Model file for the job. Use its own axes, mm. Face numbers are marked on the shaded views. A direction names the side the tool comes from. Round coordinates to 2 decimals unless told otherwise and drop trailing zeros. Loops run counter-clockwise (first coordinate to the right, second up) from the corner with the lowest first, then second, coordinate; pieces in that order, holes last. Notation, with made-up numbers: (60, 18) -> (112, 18) arc R17 ccw to (112, 51) -> close; hole circle Ø11 at (-7, -21). An arc over 180 degrees is marked (long way). Use a Markdown table: item, result.
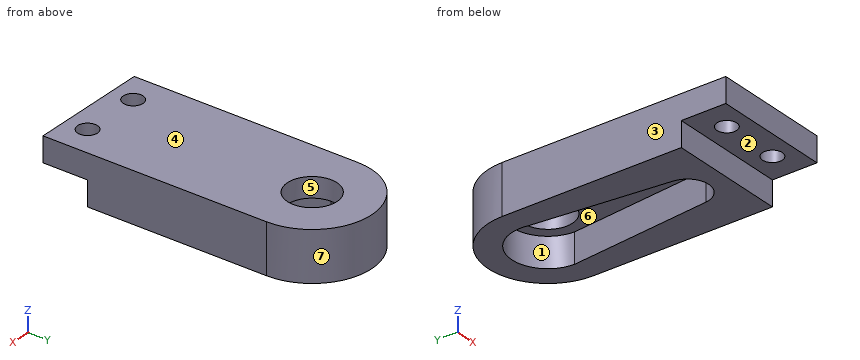
from build123d import *

# Parameters (mm, degrees)
SKETCH1_W           = 11.999998241
SKETCH1_H           = 22.605046118
BOSS_EXTRUDE1_DEPTH = 5
BOSS_EXTRUDE2_DEPTH = 5
SKETCH4_R           = 2.5
CUT_EXTRUDE3_DEPTH  = 5
CUT_EXTRUDE7_DEPTH  = 3
SKETCH10_W          = 11.999998241
SKETCH10_H          = 4.5
CUT_EXTRUDE8_DEPTH  = 2.5
SKETCH12_R          = 1
CUT_EXTRUDE9_DEPTH  = 5


with BuildPart() as part:
    # Sketch1 → Boss-Extrude1 (new body)
    with BuildSketch(Plane.XY):
        with Locations((-37.429383025, 291.690953332)):
            Rectangle(SKETCH1_W, SKETCH1_H)
    extrude(amount=BOSS_EXTRUDE1_DEPTH)

    # Sketch3 → Boss-Extrude2 (add)
    with BuildSketch(Plane.XY):
        with BuildLine():
            Line((-31.429383904, 302.993476391), (-43.429382145, 302.993476391))
            ThreePointArc((-43.429382145, 302.993476391), (-37.429383025, 308.993475512), (-31.429383904, 302.993476391))
        make_face()
    extrude(amount=BOSS_EXTRUDE2_DEPTH)

    # Sketch4 → Cut-Extrude3 (cut)
    with BuildSketch(Plane.XY):
        with Locations((-37.429383025, 302.993476391)):
            Circle(SKETCH4_R)
    extrude(amount=CUT_EXTRUDE3_DEPTH, mode=Mode.SUBTRACT)

    # Sketch6 → Cut-Extrude7 (cut)
    with BuildSketch(Plane.XY):
        with BuildLine():
            Line((-33.809082583, 303.064405918), (-35.29156372, 288.661777973))
            ThreePointArc((-35.29156372, 288.661777973), (-37.429381162, 286.732713757), (-39.567198604, 288.661777973))
            Line((-39.567198604, 288.661777973), (-40.961969567, 302.198216304))
            ThreePointArc((-40.961969567, 302.198216304), (-37.864692735, 306.588210281), (-33.809082583, 303.064405918))
        make_face()
    extrude(amount=CUT_EXTRUDE7_DEPTH, mode=Mode.SUBTRACT)

    # Sketch10 → Cut-Extrude8 (cut)
    with BuildSketch(Plane.XY):
        with Locations((-37.429383025, 282.638430273)):
            Rectangle(SKETCH10_W, SKETCH10_H)
    extrude(amount=CUT_EXTRUDE8_DEPTH, mode=Mode.SUBTRACT)

    # Sketch12 → Cut-Extrude9 (cut)
    with BuildSketch(Plane.XY):
        with Locations((-34.429383904, 282.588430273)):
            Circle(SKETCH12_R)
        with Locations((-40.429382145, 282.588430273)):
            Circle(SKETCH12_R)
    extrude(amount=CUT_EXTRUDE9_DEPTH, mode=Mode.SUBTRACT)


solid = part.part
Q1. Flat gauge pins, fed straight in: pin 1 (6 mm diameter, centred on x = -37.43, y = 302.99, fed in from +Z); pin 2 (4.5 mm diameter, centred on x = -37.43, y = 302.99, fed in from -Z); pin 3 (2.5 mm diameter, centred on x = -34.43, y = 282.59, fed in from -Z); pin 4 (1 mm diameter, centred on y = 305, z = 1.5, fed in from -X). Where does each tip first touch, or does it go through?
Results list:
| item | result |
|---|---|
| pin 1 | stops at z = 5 |
| pin 2 | passes through |
| pin 3 | stops at z = 2.5 |
| pin 4 | stops at x = -43.24 |
Q2. Band-saw the part on D-D, the plane z = 4.65. Give the cut face in (x, y).
Results list:
| item | result |
|---|---|
| outline | (-43.43, 280.39) -> (-31.43, 280.39) -> (-31.43, 302.99) arc R6 ccw to (-43.43, 302.99) -> close; hole circle Ø2 at (-40.43, 282.59); hole circle Ø5 at (-37.43, 302.99); hole circle Ø2 at (-34.43, 282.59) |
Q3. Drill centre lines: L1, parallel to X at y = 282.25, z = 3.4; L2, parallel to Y at x = -37.5, z = 0.5; L3, parallel to Z at x = -37.5, y = 294. Where is each one in solid material? Low to high. Write a range as from..to.
Results list:
| item | result |
|---|---|
| L1 | x = -43.43..-41.37, -39.49..-35.37, -33.49..-31.43 |
| L2 | y = 284.89..286.73, 306.61..308.99 |
| L3 | z = 3..5 |
Q4. Band-saw the part on C-C, the plane y = 293.5. Give the cut face in (x, z).
Results list:
| item | result |
|---|---|
| outline | (-43.43, 0) -> (-40.07, 0) -> (-40.07, 3) -> (-34.79, 3) -> (-34.79, 0) -> (-31.43, 0) -> (-31.43, 5) -> (-43.43, 5) -> close |
Q5. Pull direction X, two halves, no side cores. Call the marked faces 4, 5, 6 and 7: released by +X, released by -X, zero draft, split by the parting line, or undercut.
Results list:
| item | result |
|---|---|
| face 4 | zero draft |
| face 5 | undercut |
| face 6 | undercut |
| face 7 | split by the parting line |
Q6. Band-saw the part on B-B, the plane x = -35.75. Give the cut face in (y, z).
Results list:
| item | result |
|---|---|
| outline | (280.39, 2.5) -> (284.89, 2.5) -> (284.89, 0) -> (287.54, 0) -> (287.54, 3) -> (301.14, 3) -> (301.14, 5) -> (280.39, 5) -> close; (304.85, 3) -> (306.2, 3) -> (306.2, 0) -> (308.75, 0) -> (308.75, 5) -> (304.85, 5) -> close |
Q7. Tool access for the marked faces 1, 2 and 3: list every direction of +Z, -Z, +X, -X, +Y, -Y with a clear straight run to the whole face (end or side of a thin tool).
Results list:
| item | result |
|---|---|
| face 1 | -Z |
| face 2 | -Z, +X, -X, -Y |
| face 3 | +Z, -Z, -X, +Y, -Y |
Q8. Band-saw the part on A-A, the plane z = 1.6. Give the cut face in (x, y).
Results list:
| item | result |
|---|---|
| outline | (-43.43, 284.89) -> (-31.43, 284.89) -> (-31.43, 302.99) arc R6 ccw to (-43.43, 302.99) -> close; hole (-40.96, 302.2) -> (-39.57, 288.66) arc R2.15 ccw to (-35.29, 288.66) -> (-33.81, 303.06) arc R3.62 ccw (long way) to start |
